Source: CAD feature listing. Evaluate the final solid. Frame: model axes, mm. Give positions to 0.01 mm unless a question says otherwise; leave off trailing zeros. Loops run counter-clockwise (first coordinate to the right, second up) from the corner with the lowest first, then second, coordinate; pieces in that order, holes last. Notation, with made-up numbers: (78, 29.25) - (113, 29.25) arc R17 cw to (113, 49.25) - close; hole circle Ø5 at (73.5, 36.25). An arc over 180 degrees is marked (long way). Write each question's results on one line, items separated by ' | '. Start each with the question number.
(1) Cut plane B-B on x = -82.5. Return the cut outline in (y, z).
(2) Cut plane C-C on y = -0.9. Return the cut outline in (x, z).
(3) Material intervals for line 1 along Z through (x, y) = (-16.5, -1.75); line 2 along X through (y, z) = (-0.55, 26), sorted ascending. Write a range as [from, to].
(4) Cut plane A-A on z = -34. Return the cut outline in (x, y).
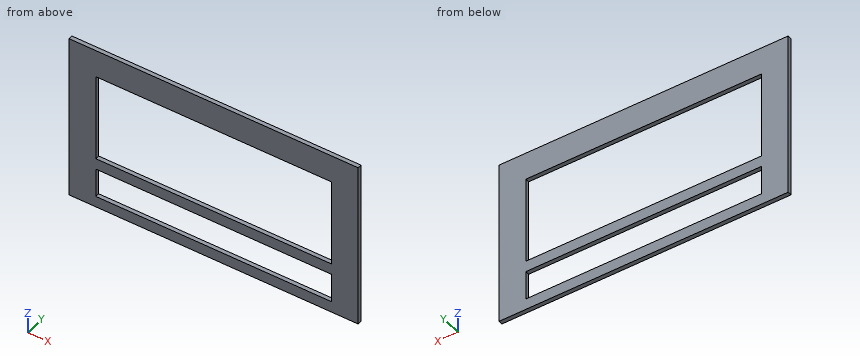
from build123d import *

# Parameters (mm, degrees)
F0_W     = 210
F0_H     = 120
F0_W_2   = 171
F0_H_2   = 21
F0_H_3   = 63
F1_DEPTH = 3


with BuildPart() as f1:
    # F0 (on Front) → F1 (new body)
    with BuildSketch(Plane.XZ):
        Rectangle(F0_W, F0_H)
        with Locations((0, -41.5)):
            Rectangle(F0_W_2, F0_H_2, mode=Mode.SUBTRACT)
        with Locations((0, 8.5)):
            Rectangle(F0_W_2, F0_H_3, mode=Mode.SUBTRACT)
    extrude(amount=F1_DEPTH)


solid = f1.part
Ans:
1) outline: (-3, -60) - (0, -60) - (0, -52) - (-3, -52) - close; (-3, -31) - (0, -31) - (0, -23) - (-3, -23) - close; (-3, 40) - (0, 40) - (0, 60) - (-3, 60) - close
2) outline: (-105, -60) - (105, -60) - (105, 60) - (-105, 60) - close; hole (-85.5, -52) - (85.5, -52) - (85.5, -31) - (-85.5, -31) - close; hole (-85.5, -23) - (85.5, -23) - (85.5, 40) - (-85.5, 40) - close
3) line 1: [-60, -52], [-31, -23], [40, 60] | line 2: [-105, -85.5], [85.5, 105]
4) outline: (-105, -3) - (-85.5, -3) - (-85.5, 0) - (-105, 0) - close; (85.5, -3) - (105, -3) - (105, 0) - (85.5, 0) - close
